from build123d import *

# Parameters (mm, degrees)
SKETCH_2_R               = 2.5
CUT_EXTRUDE_1_DEPTH      = 61.932339525
HOLE_WIZARD_M2_5_5_D     = 2.05
HOLE_WIZARD_M2_5_5_DEPTH = 18.35
HOLE_WIZARD_M2_5_5_TIP   = 0.615882135
CHAMFER_1_SIZE           = 0.5
CUT_EXTRUDE_START        = -9
SKETCH_20_R              = 3
SKETCH_20_R_2            = 2.5
CUT_EXTRUDE_6_DEPTH      = 9
HOLE_WIZARD_M3_2_D       = 2.5
HOLE_WIZARD_M3_2_DEPTH   = 18.5
HOLE_WIZARD_M3_2_TIP     = 0.751075774
SKETCH_25_R              = 28
SKETCH_25_R_2            = 26
EXTRUDE_1_DEPTH          = 1
FILLET_1_R               = 1


with BuildPart() as part:
    # Sketch 1 → Revolve 1 (revolve)
    with BuildSketch(Plane.XY, mode=Mode.PRIVATE) as revolve_1_sk:
        Polygon((26, -11.5), (26, -36.5), (34.5, -36.5), (34.5, -26), (29.5, -26), (29.5, -19.9), (27.5, -19.9), (27.5, -2.9), (26, -2.9), (26, 0), (13, 0), (13, -3), (15.5, -3), (15.5, -4.5), (17.5, -4.5), (17.5, -11.5), align=None)
    revolve(revolve_1_sk.sketch.rotate(Axis((0, 53.635658915, 0), (0, -1, 0)), 90), axis=Axis((0, 53.635658915, 0), (0, -1, 0)))

    # Sketch 2 → Cut-Extrude 1 (cut, through all)
    with BuildSketch(Plane(origin=(0, 0, 0), x_dir=(1, 0, 0), z_dir=(0, 1, 0))):
        with Locations(Location((0, 18.9, 0), (0, 0, 270))):
            Circle(SKETCH_2_R)
        with Locations(Location((-16.367880132, -9.45, 0), (0, 0, 270))):
            Circle(SKETCH_2_R)
        with Locations(Location((16.367880132, -9.45, 0), (0, 0, 270))):
            Circle(SKETCH_2_R)
    extrude(amount=-CUT_EXTRUDE_1_DEPTH, mode=Mode.SUBTRACT)

    # Hole Wizard M2.5 _5
    with Locations(Plane(origin=(-19.485571585, 0, -11.25), x_dir=(0, 0, 1), z_dir=(0, 1, 0))):
        with Locations((0, 0), (0, 38.97114317), (33.75, 19.485571585)):
            Hole(HOLE_WIZARD_M2_5_5_D / 2, depth=HOLE_WIZARD_M2_5_5_DEPTH)
            with Locations((0, 0, -(HOLE_WIZARD_M2_5_5_DEPTH + HOLE_WIZARD_M2_5_5_TIP / 2))):  # 118° drill point
                Cone(0, HOLE_WIZARD_M2_5_5_D / 2, HOLE_WIZARD_M2_5_5_TIP, mode=Mode.SUBTRACT)

    # Chamfer 1
    chamfer_1_edges = [part.edges().sort_by_distance(p)[0] for p in [
        (0, -2.9, -27.5),
        (0, 0, -26),
    ]]
    chamfer(chamfer_1_edges, length=CHAMFER_1_SIZE)

    # Sketch 20 → Cut-Extrude 6 (cut)
    # profile 1 of 3: a face of its own
    with BuildSketch(Plane.XZ.offset(11.5).offset(CUT_EXTRUDE_START)):
        with Locations(Location((-16.367880132, 9.45, 0), (0, 0, 270))):
            Circle(SKETCH_20_R)
        with Locations(Location((-16.367880132, 9.45, 0), (0, 0, 90))):
            Circle(SKETCH_20_R_2, mode=Mode.SUBTRACT)
    # profile 2 of 3: a face of its own
    with BuildSketch(Plane.XZ.offset(11.5).offset(CUT_EXTRUDE_START)):
        with Locations(Location((16.367880132, 9.45, 0), (0, 0, 270))):
            Circle(SKETCH_20_R)
        with Locations(Location((16.367880132, 9.45, 0), (0, 0, 90))):
            Circle(SKETCH_20_R_2, mode=Mode.SUBTRACT)
    # profile 3 of 3: a face of its own
    with BuildSketch(Plane.XZ.offset(11.5).offset(CUT_EXTRUDE_START)):
        with Locations(Location((0, -18.9, 0), (0, 0, 270))):
            Circle(SKETCH_20_R)
        with Locations(Location((0, -18.9, 0), (0, 0, 90))):
            Circle(SKETCH_20_R_2, mode=Mode.SUBTRACT)
    extrude(amount=CUT_EXTRUDE_6_DEPTH, mode=Mode.SUBTRACT)

    # Hole Wizard M3 _2
    with Locations(Plane(origin=(0, -26, 0), x_dir=(1, 0, 0), z_dir=(0, 1, 0))):
        with Locations((-27.712812921, 16), (-27.712812921, -16), (0, -32), (27.712812921, -16), (27.712812921, 16), (0, 32)):
            Hole(HOLE_WIZARD_M3_2_D / 2, depth=HOLE_WIZARD_M3_2_DEPTH)
            with Locations((0, 0, -(HOLE_WIZARD_M3_2_DEPTH + HOLE_WIZARD_M3_2_TIP / 2))):  # 118° drill point
                Cone(0, HOLE_WIZARD_M3_2_D / 2, HOLE_WIZARD_M3_2_TIP, mode=Mode.SUBTRACT)

    # Sketch 25 → Extrude 1 (add)
    with BuildSketch(Plane.XZ.offset(36.5)):
        with Locations(Location((0, 0, 0), (0, 0, 90))):
            Circle(SKETCH_25_R)
        with Locations(Location((0, 0, 0), (0, 0, 90))):
            Circle(SKETCH_25_R_2, mode=Mode.SUBTRACT)
    extrude(amount=EXTRUDE_1_DEPTH)

    # Fillet 1
    # the kernel refuses this fillet: 1 mm, written as the material it takes off along each edge
    with BuildSketch(Plane(origin=(-16.267321543, -4.5, 6.451685812), x_dir=(-0.33722091100781637, 0, -0.9414255452127154), z_dir=(0, -1, 0)), Plane(origin=(2.546336961, -4.5, -17.313756614), x_dir=(0.9839088934297354, 0, 0.1786708969862573), z_dir=(0, -1, 0))) as fillet_1_piece_1:
        with BuildLine():
            CenterArc((1.209807448, -0.999435167), FILLET_1_R, 91.92583096, 89.597377695)
            ThreePointArc((0.210160808, -1.026017042), (0.150200412, -0.503766513), (0, 0))
            ThreePointArc((0, 0), (0.588100843, -0.00988458), (1.176201685, 0))
        make_face()
    extrude(amount=9.940504213, mode=Mode.SUBTRACT)
    with BuildSketch(Plane(origin=(-13.720984582, -4.5, 10.862070802), x_dir=(-0.6174722047183601, 0, 0.7865927004493796), z_dir=(0, -1, 0)), Plane(origin=(16.267321543, -4.5, 6.451685812), x_dir=(0.989945363379746, 0, 0.1414502651921957), z_dir=(0, -1, 0)), Plane(origin=(-2.546336961, -4.5, -17.313756614), x_dir=(-0.3724731586613872, 0, -0.9280429656415747), z_dir=(0, -1, 0))) as fillet_1_piece_2:
        with BuildLine():
            CenterArc((1.221872973, -0.98464773), FILLET_1_R, 100.052662926, 89.597377695)
            ThreePointArc((0.236022963, -1.152277556), (0.127695008, -0.574155285), (0, 0))
            ThreePointArc((0, 0), (0.523659845, -0.046056811), (1.047319691, 0))
        make_face()
    extrude(amount=9.940504213, mode=Mode.SUBTRACT)
    with BuildSketch(Plane(origin=(13.720984582, -4.5, 10.862070802), x_dir=(0.6174722047183601, 0, 0.7865927004493796), z_dir=(0, -1, 0))) as fillet_1_piece_3:
        with BuildLine():
            CenterArc((1.221872973, 0.98464773), FILLET_1_R, 170.349959378, 89.597377695)
            ThreePointArc((0.236022963, 1.152277556), (0.127695008, 0.574155285), (0, 0))
            ThreePointArc((0, 0), (0.523659845, 0.046056811), (1.047319691, 0))
        make_face()
    extrude(amount=9.940504213, mode=Mode.SUBTRACT)


solid = part.part
Design review of the part built by this model. Coordinates are the model's own, in mm. A direction names the side the tool comes from. Coordinates: 2 decimals unless noted, no trailing zeros. Order: outer loops, then holes, each group sorted by start corner. A loop starts at its lowest first (then second) coordinate and runs counter-clockwise, first axis right, second up. Notation, with made-up numbers: M 68.5,-32 L 116.5,-32 A25 ccw 116.5,-16 Z; hole C -35.75,59 d10. An arc over 180 degrees is marked long. Use a Markdown table: item, result.
(1) Wall thickness on probe 1 along X at (y, z) = (-1.65, 9.45); probe 2 along X at (y, z) = (-33.25, 16); probe 3 along Y at (x, z) = (-18, -8): over which ranges is each line inside the solid? List them lowest first.
Worked answers:
| item | result |
|---|---|
| probe 1 | x = -24.22 to -18.87, -13.87 to -8.93, 8.93 to 13.87, 18.87 to 24.22 |
| probe 2 | x = -30.57 to -28.96, -26.46 to -20.49, 20.49 to 26.46, 28.96 to 30.57 |
| probe 3 | y = -11.5 to 0 |
(2) For faces 4 (the flat face through (-14, -2.5, 11)), 5 (the cylindrical face through (-0.577, -31.323, 33.109)), 6 (the flat face through (20, -19.9, 20)), list the 3-axis set-ups (+Z, -Z, +X, -X, +Y, -Y) from which the entire face can be reached by the end or side of a thin tool; tool diameter is ignored.
Worked answers:
| item | result |
|---|---|
| face 4 | -Y |
| face 5 | +Y, -Y |
| face 6 | +Y |
(3) Add section B-B (z = -32). Give the boundary of the cut face in (x, y), then the cut area to 3 significant figures.
Worked answers:
| item | result |
|---|---|
| outline | M -12.89,-36.5 L -1.25,-36.5 L -1.25,-26 L -12.89,-26 Z; M 1.25,-36.5 L 12.89,-36.5 L 12.89,-26 L 1.25,-26 Z |
| area | 245 mm2 |
(4) Add section D-D (y = -19). Give the boundary of the cut face in (x, z).
Worked answers:
| item | result |
|---|---|
| outline | C 0,0 d55; hole C 0,0 d52 |
(5) Add section C-C (x = 0). Count the separate pieces of the cut face and the enclosed holes in it, then the cut area to 3 significant figures.
Worked answers:
| item | result |
|---|---|
| separate pieces | 6 |
| enclosed holes | 0 |
| area | 373 mm2 |
(6) Draft analysis for pull direction Z (two halves, no side actions). For faces 1 (the cylindrical face through (24.397, -11.534, 12.69)), 2 (the flat face through (28, -36.5, -5)), 3 (the flat face through (2, -2.5, -17)), state which applies: released by +Z, released by -Z, zero draft, split by the parting line, or undercut.
Worked answers:
| item | result |
|---|---|
| face 1 | split by the parting line |
| face 2 | zero draft |
| face 3 | undercut |
(7) For P1, Ø6, axis at x = -3.5, y = -7.5, coming from the -Z side; P2, Ø8, axis at x = -11, y = -21.5, coming from the -Z side; P3, Ø1.8, axis at x = 19.49, z = -11.25, coming from the -Y side; P4, Ø3, axis at x = 27.71, z = 16, coming from the -Y side, all flat-tipped, find the tip position at first contact; note any pin that passes through.
Worked answers:
| item | result |
|---|---|
| P1 | stops at z = -27.5 |
| P2 | stops at z = -28.66 |
| P3 | passes through |
| P4 | stops at y = -36.5 |
(8) Add section A-A (y = -27.5). Give the boundary of the cut face in (x, z).
Worked answers:
| item | result |
|---|---|
| outline | C 0,0 d69; hole C -27.71,-16 d2.5; hole C -27.71,16 d2.5; hole C 0,0 d52; hole C 0,-32 d2.5; hole C 0,32 d2.5; hole C 27.71,-16 d2.5; hole C 27.71,16 d2.5 |
